Read the model definition and answer for the solid it produces. Units are mm, in the model's axes. A direction names the side the tool comes from. Round coordinates to 2 decimals unless told otherwise and drop trailing zeros. Order: outer loops, then holes, each group sorted by start corner. A loop starts at its lowest first (then second) coordinate and runs counter-clockwise, first axis right, second up. Notation, with made-up numbers: (23, 84.5) -> (56, 84.5) arc R7 ccw to (56, 88.5) -> close; hole circle Ø10 at (29, 22). An arc over 180 degrees is marked (long way). Use a Markdown table: item, result. Add a question column.
1. Section C-C, the plane z = 22.5 is taken. Give the vertices of the cut face in (x, y), then the cut area to 3 significant figures.
2. Given pin 1 (6 mm diameter, centred on x = 25, z = 6, fed in from -Y); pin 2 (5 mm diameter, centred on x = 19.5, z = -3, fed in from -Y); pin 3 (1 mm diameter, centred on x = -8.5, z = 13, fed in from +Y), each flat-ended and moving along its own axis, determine where each tip first touches the part or whether it passes through.
3. For faces 5 (the face through (-21, -5, -3)), 6 (the face through (12.5, 0, 13)), 7 (the face through (0, -16, -6)), determine the directions among +Z, -Z, +X, -X, +Y, -Y from which every point of the face is accessible in a straight line to the end or side of a thin tool.
4. Section D-D, the plane x = -22 is taken. Give the vertices of the cut face in (y, z), then the cut area to 3 significant figures.
5. Section A-A, the plane y = 0 is taken. Give the vertices of the cut face in (x, z), then the cut area to 3 significant figures.
6. Section B-B, the plane x = 0 is taken. Give the vertices of the cut face in (y, z), then the cut area to 3 significant figures.
7. The mould has two halves that part along Y. Classify faces 1 (the face through (-4.336, -19.524, 15.86)), 2 (the face through (11, 2.5, 13)), 3 (the face through (22, 0, 0)), 4 (the face through (15, -15, 6)): +Y half, -Y half, draft (parallel to the pull), parting line (faces both ways), or undercut.
8. Consider L1, parallel to Y at x = 0, z = 3.5; L2, parallel to Y at x = 0, z = 6.5; L3, parallel to Z at x = 5.5, y = -21. Determine where each line is inside the solid, lowest interval first. Write a range as [from, to].
```python
from build123d import *

# Parameters (mm, degrees)
SKETCH1_R           = 35
BOSS_EXTRUDE1_DEPTH = 6
SKETCH2_R           = 20
SKETCH2_R_2         = 10
BOSS_EXTRUDE2_DEPTH = 20
CUT_EXTRUDE1_START  = -20
SKETCH3_R           = 10
CUT_EXTRUDE1_DEPTH  = 20
SKETCH4_W           = 5
SKETCH4_H           = 5
CUT_EXTRUDE2_DEPTH  = 59.940648113
SKETCH5_W           = 82.032874524
SKETCH5_H           = 10
CUT_EXTRUDE3_DEPTH  = 6


with BuildPart() as part:
    # Sketch1 → Boss-Extrude1 (new, symmetric)
    with BuildSketch(Plane.XY):
        Circle(SKETCH1_R)
    extrude(amount=BOSS_EXTRUDE1_DEPTH, both=True)

    # Sketch2 → Boss-Extrude2 (add)
    with BuildSketch(Plane.XY.offset(6)):
        Circle(SKETCH2_R)
        Circle(SKETCH2_R_2, mode=Mode.SUBTRACT)
    extrude(amount=BOSS_EXTRUDE2_DEPTH)

    # Sketch3 → Cut-Extrude1 (cut)
    with BuildSketch(Plane.XY.offset(6).offset(CUT_EXTRUDE1_START)):
        Circle(SKETCH3_R)
    extrude(amount=CUT_EXTRUDE1_DEPTH, mode=Mode.SUBTRACT)

    # Sketch4 → Cut-Extrude2 (cut, through all)
    with BuildSketch(Plane.XY.offset(26)):
        with Locations((10, 0)):
            Rectangle(SKETCH4_W, SKETCH4_H)
    extrude(amount=-CUT_EXTRUDE2_DEPTH, mode=Mode.SUBTRACT)

    # Sketch5 → Cut-Extrude3 (cut)
    with BuildSketch(Plane(origin=(0, 0, -6), x_dir=(-1, 0, 0), z_dir=(0, 0, -1))):
        Rectangle(SKETCH5_W, SKETCH5_H)
    extrude(amount=-CUT_EXTRUDE3_DEPTH, mode=Mode.SUBTRACT)


solid = part.part
```
Verdict:
| question | item | result |
|---|---|---|
| 1 | outline | circle Ø40 at (0, 0); hole (9.68, -2.5) -> (12.5, -2.5) -> (12.5, 2.5) -> (9.68, 2.5) arc R10 ccw (long way) to start |
| 1 | area | 929 mm2 |
| 2 | pin 1 | stops at y = -27.22 |
| 2 | pin 2 | stops at y = -30.59 |
| 2 | pin 3 | stops at y = 18.33 |
| 3 | face 5 | -Z, +X, -X |
| 3 | face 6 | +Z, -Z |
| 3 | face 7 | -Z, +X, -X, +Y, -Y |
| 4 | outline | (-27.22, -6) -> (-5, -6) -> (-5, 0) -> (5, 0) -> (5, -6) -> (27.22, -6) -> (27.22, 6) -> (-27.22, 6) -> close |
| 4 | area | 593 mm2 |
| 5 | outline | (-35, 0) -> (-10, 0) -> (-10, 26) -> (-20, 26) -> (-20, 6) -> (-35, 6) -> close; (12.5, 0) -> (35, 0) -> (35, 6) -> (20, 6) -> (20, 26) -> (12.5, 26) -> close |
| 5 | area | 635 mm2 |
| 6 | outline | (-35, -6) -> (-10, -6) -> (-10, 26) -> (-20, 26) -> (-20, 6) -> (-35, 6) -> close; (10, -6) -> (35, -6) -> (35, 6) -> (20, 6) -> (20, 26) -> (10, 26) -> close |
| 6 | area | 1,000 mm2 |
| 7 | face 1 | parting line |
| 7 | face 2 | undercut |
| 7 | face 3 | undercut |
| 7 | face 4 | draft |
| 8 | L1 | y = [-35, -10], [10, 35] |
| 8 | L2 | y = [-20, -10], [10, 20] |
| 8 | L3 | z = [-6, 6] |
